```python
from build123d import *

# Parameters (mm, degrees)
SKETCH1_W               = 25
SKETCH1_H               = 38.5
SKETCH1_H_2             = 1.5
BOSS_EXTRUDE1_DEPTH     = 1.5
SKETCH1_3_W             = 25
SKETCH1_3_H             = 1.5
BOSS_EXTRUDE2_DEPTH     = 30
FILLET1_R               = 12.5
SKETCH2_R               = 2.5
CUT_EXTRUDE1_DEPTH      = 39.160843806
CUT_EXTRUDE2_DEPTH      = 51.383529055
CUT_EXTRUDE2_DEPTH_BACK = 51.383529055
SKETCH3_R               = 2.5


with BuildPart() as part:
    # Sketch1 → Boss-Extrude1 (new body)
    with BuildSketch(Plane(origin=(0, 0, 0), x_dir=(1, 0, 0), z_dir=(0, 1, 0))):
        with Locations((0, 0.75)):
            Rectangle(SKETCH1_W, SKETCH1_H)
        with Locations((0, -19.25)):
            Rectangle(SKETCH1_W, SKETCH1_H_2)
    extrude(amount=-BOSS_EXTRUDE1_DEPTH)

    # Sketch1<3> → Boss-Extrude2 (add)
    with BuildSketch(Plane(origin=(0, 0, 0), x_dir=(1, 0, 0), z_dir=(0, 1, 0))):
        with Locations((0, -19.25)):
            Rectangle(SKETCH1_3_W, SKETCH1_3_H)
    extrude(amount=BOSS_EXTRUDE2_DEPTH)

    # Fillet1
    fillet1_edges = [part.edges().sort_by_distance(p)[0] for p in [
        (-12.5, 30, 19.25),
        (12.5, 30, 19.25),
        (-12.5, -0.75, -20),
        (12.5, -0.75, -20),
    ]]
    fillet(fillet1_edges, radius=FILLET1_R - 0.0001)  # a hair under: the kernel refuses the full size

    # Sketch2 → Cut-Extrude1 (cut, through all)
    with BuildSketch(Plane(origin=(0, 0, 0), x_dir=(1, 0, 0), z_dir=(0, 1, 0))):
        with Locations(Location((0, 7.5, 0), (0, 0, 270))):
            Circle(SKETCH2_R)
    extrude(amount=-CUT_EXTRUDE1_DEPTH, mode=Mode.SUBTRACT)

    # Sketch3 → Cut-Extrude2 (cut, two sides: drawn at the far end of the back side and taken through both)
    with BuildSketch(Plane(origin=(0, 0, 18.5), x_dir=(-1, 0, 0), z_dir=(0, 0, -1)).offset(-CUT_EXTRUDE2_DEPTH_BACK)):
        with Locations((0, 17.5)):
            Circle(SKETCH3_R)
    extrude(amount=CUT_EXTRUDE2_DEPTH + CUT_EXTRUDE2_DEPTH_BACK, mode=Mode.SUBTRACT)


solid = part.part
```
The listing builds one solid part. Answer for the finished solid, in the listing's coordinates (mm). A direction names the side the tool comes from. Round coordinates to 2 decimals unless told otherwise and drop trailing zeros. Write each loop counter-clockwise with the first axis right and the second up, starting at its lowest first coordinate (ties: lowest second). Pieces come first, ordered by that corner, then holes. Notation, with made-up numbers: (11, 20.5) -> (68, 20.5) arc R17 cw to (68, 28.5) -> close; hole circle Ø2 at (9.25, 30). An arc over 180 degrees is marked (long way). Write item = value, one per line.
1) For a pull along X with two mould halves and no side action, classify faces 1 (the flat face through (-12.5, -0.5, 12.4)), 2 (the cylindrical face through (-1.34, 19.61, 19.26)), 3 (the flat face through (0, 0, -1)) as released by +X, released by -X, zero draft, split by the parting line, or undercut.
Check values:
face_1 = released by -X
face_2 = undercut
face_3 = zero draft
2) Given pin 1 (7.5 mm diameter, centred on x = -4.5, z = 0.5, fed in from +Y); pin 2 (1 mm diameter, centred on x = 3, y = 21, fed in from -Z); pin 3 (3 mm diameter, centred on x = 0, y = 17.5, fed in from -Z), each flat-ended and moving along its own axis, determine where each tip first touches the part or whether it passes through.
Check values:
pin_1 = 0
pin_2 = 18.5
pin_3 = through
3) Which of the six approach directions +Z, -Z, +X, -X, +Y, -Y give full straight-line access (tool end or side, diameter ignored) to faces 4 (the flat face through (-0.2, 14.8, 18.5)), 5 (the cylindrical face through (0, -1, -10))?
Check values:
face_4 = -Z, +X, -X, +Y
face_5 = +Y, -Y
4) Straight lines are drawn through the part: line 1 along Y through (x, z) = (0, 19.05); line 2 along X through (y, z) = (17.5, 19.35); line 3 along Z through (x, y) = (10.5, 2). For each, find the intervals that lie inside material, in ascending order. Write a range as [from, to].
Check values:
line_1 = [-1.5, 15], [20, 30]
line_2 = [-12.5, -2.5], [2.5, 12.5]
line_3 = [18.5, 20]
5) Section A-A on x = -7.75 is taken. Write down the section's boundary in (y, z).
Check values:
outline = (-1.5, -17.31) -> (0, -17.31) -> (0, 18.5) -> (27.31, 18.5) -> (27.31, 20) -> (-1.5, 20) -> close
6) Section C-C on z = -12 is taken. Write down the section's boundary in (x, y), plus the area to 3 significant figures.
Check values:
outline = (-11.66, -1.5) -> (11.66, -1.5) -> (11.66, 0) -> (-11.66, 0) -> close
area = 35.0 mm²
7) Section B-B on y = 7.5 is taken. Write down the section's boundary in (x, z).
Check values:
outline = (-12.5, 18.5) -> (12.5, 18.5) -> (12.5, 20) -> (-12.5, 20) -> close
